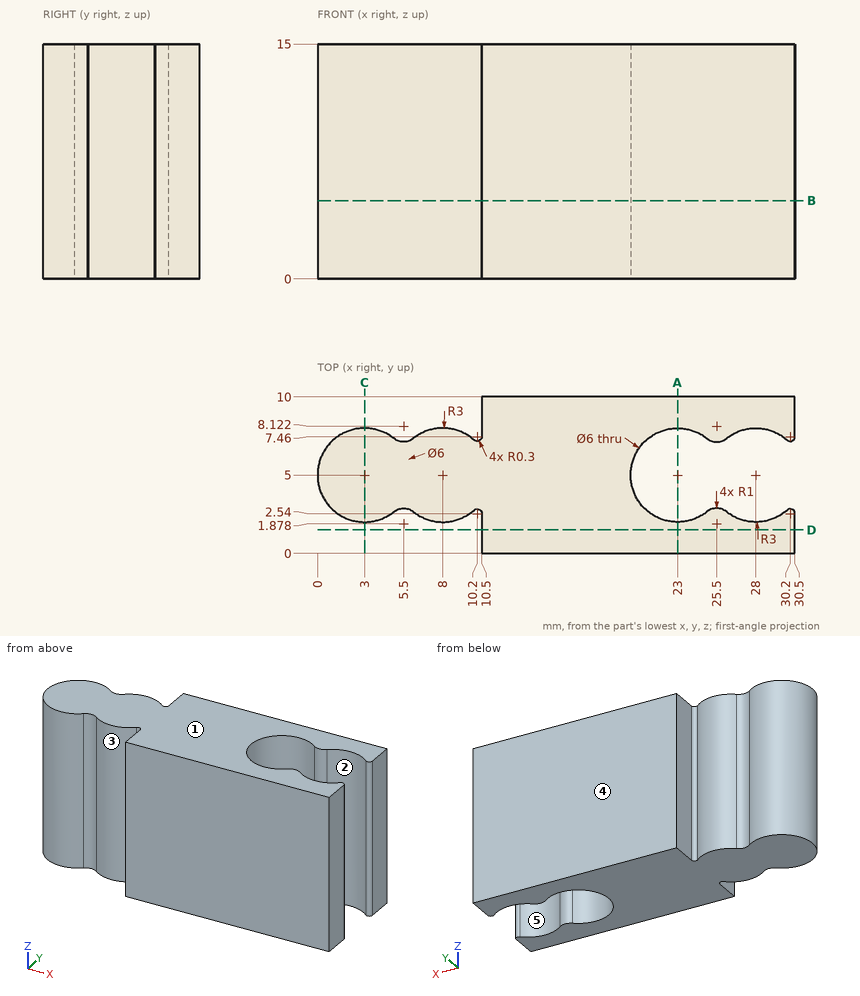
The figure shows three views and two pictorial views of one solid part (mm, origin at its lowest corner). Answer the questions. A direction names the side the tool comes from. Give positions to 0.01 mm unless a question says otherwise; leave off trailing zeros. Order: outer loops, then holes, each group sorted by start corner. A loop starts at its lowest first (then second) coordinate and runs counter-clockwise, first axis right, second up. Notation, with made-up numbers: M 67,82.25 L 81,82.25 A25 cw 81,106.25 Z; hole C 87,-0.5 d5. An arc over 180 degrees is marked long. Return JSON: item names as keys, results as strings.
1) Section B-B, the plane z = 5 is taken. Write down the section's boundary in (x, y) (1 decimal).
Resolved:
{"outline": "M 4.9,2.7 A1 cw 6.1,2.7 A3 ccw 10,2.8 A0.3 cw 10.5,2.5 L 10.5,0 L 30.5,0 L 30.5,2.5 A0.3 ccw 30,2.8 A3 cw 26.1,2.7 A1 ccw 24.9,2.7 A3 cw long 24.9,7.3 A1 ccw 26.1,7.3 A3 cw 30,7.2 A0.3 ccw 30.5,7.5 L 30.5,10 L 10.5,10 L 10.5,7.5 A0.3 cw 10,7.2 A3 ccw 6.1,7.3 A1 cw 4.9,7.3 A3 ccw long Z"}
2) Section D-D, the plane y = 1.5 is taken. Write down the section's boundary in (x, z), plus the area to 3 significant figures.
Resolved:
{"outline": "M 10.5,0 L 30.5,0 L 30.5,15 L 10.5,15 Z", "area": "300 mm^2"}
3) Straight lines are drawn through the part: line 1 along Y through (x, z) = (23, 7.25); line 2 along X through (y, z) = (2.75, 8.25) (1 decimal); line 3 along Y through (x, z) = (1, 1.75) (1 decimal). For each, find the intervals that lie inside material, in ascending order. Write a range as [from, to].
Resolved:
{"line 1": "[0, 2], [8, 10]", "line 2": "[1, 5], [6, 10], [10.4, 21], [25, 26], [30, 30.4]", "line 3": "[2.8, 7.2]"}
4) Each of these flat-tipped pins is pushed along its axis until it touches: pin 1 (4 mm diameter, centred on y = 5.5, z = 13, fed in from -X); pin 2 (0.8 mm diameter, centred on y = 1.5, z = 4, fed in from -X). Where does it stop, or does it pass through?
Resolved:
{"pin 1": "x = 0", "pin 2": "x = 10.5"}
5) Section A-A, the plane x = 23 is taken. Write down the section's boundary in (y, z).
Resolved:
{"outline": "M 0,0 L 2,0 L 2,15 L 0,15 Z; M 8,0 L 10,0 L 10,15 L 8,15 Z"}
6) For a pull along Y with two mould halves and no side action, classify the marked faces 1, 2 and 3 as +Y half, -Y half, draft (parallel to the pull), parting line (faces both ways), or undercut.
Resolved:
{"face 1": "draft", "face 2": "undercut", "face 3": "-Y half"}
7) Section C-C, the plane x = 3 is taken. Write down the section's boundary in (y, z).
Resolved:
{"outline": "M 2,0 L 8,0 L 8,15 L 2,15 Z"}
8) A tool of negligible diameter and unlimited length cuts with its end or side. For the marked faces 4 and 5, from which of +Z, -Z, +X, -X, +Y, -Y can it reach the whole face along a straight path? Write none if from no direction.
Resolved:
{"face 4": "+Z, -Z, +X, -X, +Y", "face 5": "+Z, -Z"}
